Autodesk Inventor part; units mm, degrees
ref_plane "YZ Plane" through (0, 0, 0) normal (1, 0, 0) x (0, 1, 0)
ref_plane "XZ Plane" through (0, 0, 0) normal (0, 1, 0) x (-1, 0, 0)
ref_plane "XY Plane" through (0, 0, 0) normal (0, 0, 1) x (1, 0, 0)
sketch "Sketch1" plane through (0, 0, 0) normal (0, 0, 1) x (1, 0, 0)
  circle A0 centre (9.5, 9.5) radius 1
  arc A1 (12.2, 7.5) -> (12.5, 7.8) centre (12.2, 7.8) ccw
  line L0 (12.5, 7.8) -> (12.5, 12.2)
  arc A2 (12.5, 12.2) -> (12.2, 12.5) centre (12.2, 12.2) ccw
  line L1 (12.2, 12.5) -> (7.8, 12.5)
  arc A3 (7.8, 12.5) -> (7.5, 12.2) centre (7.8, 12.2) ccw
  line L2 (7.5, 12.2) -> (7.5, 7.8)
  arc A4 (7.5, 7.8) -> (7.8, 7.5) centre (7.8, 7.8) ccw
  line L3 (7.8, 7.5) -> (12.2, 7.5)
  circle A5 centre (9.5, -9.5) radius 1
  arc A6 (12.5, -7.8) -> (12.2, -7.5) centre (12.2, -7.8) ccw
  line L4 (12.2, -7.5) -> (7.8, -7.5)
  arc A7 (7.8, -7.5) -> (7.5, -7.8) centre (7.8, -7.8) ccw
  line L5 (7.5, -7.8) -> (7.5, -12.2)
  arc A8 (7.5, -12.2) -> (7.8, -12.5) centre (7.8, -12.2) ccw
  line L6 (7.8, -12.5) -> (12.2, -12.5)
  arc A9 (12.2, -12.5) -> (12.5, -12.2) centre (12.2, -12.2) ccw
  line L7 (12.5, -12.2) -> (12.5, -7.8)
  circle A10 centre (-9.5, -9.5) radius 1
  arc A11 (-12.2, -7.5) -> (-12.5, -7.8) centre (-12.2, -7.8) ccw
  line L8 (-12.5, -7.8) -> (-12.5, -12.2)
  arc A12 (-12.5, -12.2) -> (-12.2, -12.5) centre (-12.2, -12.2) ccw
  line L9 (-12.2, -12.5) -> (-7.8, -12.5)
  arc A13 (-7.8, -12.5) -> (-7.5, -12.2) centre (-7.8, -12.2) ccw
  line L10 (-7.5, -12.2) -> (-7.5, -7.8)
  arc A14 (-7.5, -7.8) -> (-7.8, -7.5) centre (-7.8, -7.8) ccw
  line L11 (-7.8, -7.5) -> (-12.2, -7.5)
  circle A15 centre (-9.5, 9.5) radius 1
  arc A16 (-12.5, 7.8) -> (-12.2, 7.5) centre (-12.2, 7.8) ccw
  line L12 (-12.2, 7.5) -> (-7.8, 7.5)
  arc A17 (-7.8, 7.5) -> (-7.5, 7.8) centre (-7.8, 7.8) ccw
  line L13 (-7.5, 7.8) -> (-7.5, 12.2)
  arc A18 (-7.5, 12.2) -> (-7.8, 12.5) centre (-7.8, 12.2) ccw
  line L14 (-7.8, 12.5) -> (-12.2, 12.5)
  arc A19 (-12.2, 12.5) -> (-12.5, 12.2) centre (-12.2, 12.2) ccw
  line L15 (-12.5, 12.2) -> (-12.5, 7.8)
  line L16 (9.5, 12.5) -> (-9.5, 12.5)
  line L17 (-12.5, 9.5) -> (-12.5, -9.5)
  line L18 (-9.5, -12.5) -> (9.5, -12.5)
  line L19 (12.5, -9.5) -> (12.5, 9.5)
  line L20 (12.5, 12.5) -> (-12.5, -12.5) construction
  line L21 (-12.5, 12.5) -> (12.5, -12.5) construction
  arc A20 (12.5, 9.5) -> (9.5, 12.5) centre (9.5, 9.5) ccw
  arc A21 (-9.5, 12.5) -> (-12.5, 9.5) centre (-9.5, 9.5) ccw
  arc A22 (-12.5, -9.5) -> (-9.5, -12.5) centre (-9.5, -9.5) ccw
  arc A23 (9.5, -12.5) -> (12.5, -9.5) centre (9.5, -9.5) ccw
  point P0 (0, 0)
  point P1 (0, 0)
  point P2 (-9.5, 12.5)
  point P3 (-12.5, -9.5)
  point P4 (-12.5, -9.5)
  dimension "d0" = 25
  dimension "d1" = 25
  dimension "d2" = 3
extrude "Extrusion1" add sketch "Sketch1" along normal blind 10 contours L3 A4 L2 A3 L1 A20 L0 A1 | A1 L19 A6 L4 A7 L5 A8 L18 A13 L10 A14 L11 A11 L17 A16 L12 A17 L13 A18 L16 A3 L2 A4 L3 | L7 A23 L6 A8 L5 A7 L4 A6 | A18 L13 A17 L12 A16 L15 A21 L14 | L9 A22 L8 A11 L11 A14 L10 A13
sketch "Sketch2" plane through (0, 0, 10) normal (0, 0, 1) x (1, 0, 0)
  circle A0 centre (0, 0) radius 10.5
  dimension "d5" = 21
extrude "Extrusion2" cut sketch "Sketch2" against normal blind 4
sketch "Sketch3" plane through (0, 0, 6) normal (0, 0, 1) x (1, 0, 0)
  circle A0 centre (0, 0) radius 8
  dimension "d8" = 16
extrude "Extrusion3" add sketch "Sketch3" along normal up to surface (4 mm away)
sketch "Sketch4" plane through (0, 0, 10) normal (0, 0, 1) x (1, 0, 0)
  circle A0 centre (9.5, -9.5) radius 1
  circle A1 centre (-9.5, -9.5) radius 1
  circle A2 centre (-9.5, 9.5) radius 1
  circle A3 centre (9.5, 9.5) radius 1
  circle A4 centre (9.5, -9.5) radius 2.5
  line L0 (-9.5, -12.5) -> (9.5, -12.5)
  line L1 (12.5, -9.5) -> (12.5, 9.5)
  circle A5 centre (-9.5, -9.5) radius 2.5
  circle A6 centre (9.5, 9.5) radius 2.5
  circle A7 centre (-9.5, 9.5) radius 2.5
  point P0 (0, 0)
  dimension "d11" = 5
  dimension "d12" = 19
  dimension "d13" = 19
  dimension "d16" = 19
  dimension "d19" = 19
extrude "Extrusion4" cut sketch "Sketch4" against normal blind 1 contours A0 | A1 | A2 | A3 | A4 | A5 | A6 | A7
equation "\"d16\" = d12"
equation "\"d19\" = d13"
properties part number "fan" material "Polyethylene, Low Density"
For this review, take the finished solid that the model builds, in its own axes (mm). A direction names the side the tool comes from. Coordinates: 2 decimals unless noted, no trailing zeros. Write each loop counter-clockwise with the first axis right and the second up, starting at its lowest first coordinate (ties: lowest second). Pieces come first, ordered by that corner, then holes. Notation, with made-up numbers: (-39, 11) -> (-20, 11) arc R20 ccw to (-20, 41) -> close; hole circle Ø5 at (-39, 85.25). An arc over 180 degrees is marked (long way). Write each question's results on one line, items separated by ' | '. Start each with the question number.
1) Wall thickness on L1, parallel to X at y = 9.5, z = 4; L2, parallel to Y at x = -1.75, z = 8; L3, parallel to X at y = -5, z = 6.25 (3 decimals): over which ranges is each line inside the solid? List them lowest first. Write a range as [from, to].
2) The part is to be moulded in two halves that separate along X. For faces 1 (the face through (12.5, 0, 5)), 2 (the face through (9, -11, 9)), 3 (the face through (0, 0, 10)), say which applies: +X half, -X half, draft (parallel to the pull), parting line (faces both ways), or undercut.
3) Insertion check: pin 1 (4.5 mm diameter, centred on x = -9.5, y = -9.5, fed in from +Z); pin 2 (1.8 mm diameter, centred on x = 9.5, y = 9.5, fed in from -Z). Each pin has a flat end and moves straight along its axis. Give the tip position at first contact, or say it passes through.
4) Consider section C-C (y = 2.5). Write out the cut boundary in (x, z), plus the area to 3 significant figures.
5) For faces 4 (the face through (-10.04, 7.06, 9.51)), 5 (the face through (0, -12.5, 5)), list the 3-axis set-ups (+Z, -Z, +X, -X, +Y, -Y) from which the entire face can be reached by the end or side of a thin tool; tool diameter is ignored.
6) Consider section A-A (z = 6.75). Write out the cut boundary in (x, y).
7) Consider section B-B (x = 0). Write out the cut boundary in (y, z), plus the area to 3 significant figures.
Geometry says:
1) L1: [-12.5, -10.5], [-8.5, 8.5], [10.5, 12.5] | L2: [-12.5, -10.35], [-7.81, 7.81], [10.35, 12.5] | L3: [-12.5, -9.233], [-6.245, 6.245], [9.233, 12.5]
2) face 1: +X half | face 2: undercut | face 3: draft
3) pin 1: z = 9 | pin 2: through
4) outline: (-12.5, 0) -> (12.5, 0) -> (12.5, 10) -> (10.2, 10) -> (10.2, 6) -> (7.6, 6) -> (7.6, 10) -> (-7.6, 10) -> (-7.6, 6) -> (-10.2, 6) -> (-10.2, 10) -> (-12.5, 10) -> close | area: 229 mm^2
5) face 4: +Z | face 5: +Z, -Z, +X, -X, -Y
6) outline: (-12.5, -9.5) arc R3 ccw to (-9.5, -12.5) -> (9.5, -12.5) arc R3 ccw to (12.5, -9.5) -> (12.5, 9.5) arc R3 ccw to (9.5, 12.5) -> (-9.5, 12.5) arc R3 ccw to (-12.5, 9.5) -> close; circle Ø16 at (0, 0); hole circle Ø2 at (-9.5, -9.5); hole circle Ø21 at (0, 0); hole circle Ø2 at (-9.5, 9.5); hole circle Ø2 at (9.5, -9.5); hole circle Ø2 at (9.5, 9.5)
7) outline: (-12.5, 0) -> (12.5, 0) -> (12.5, 10) -> (10.5, 10) -> (10.5, 6) -> (8, 6) -> (8, 10) -> (-8, 10) -> (-8, 6) -> (-10.5, 6) -> (-10.5, 10) -> (-12.5, 10) -> close | area: 230 mm^2
